Design review of the part built by this model. Coordinates are the model's own, in mm. A direction names the side the tool comes from. Coordinates: 2 decimals unless noted, no trailing zeros. Write each loop counter-clockwise with the first axis right and the second up, starting at its lowest first coordinate (ties: lowest second). Pieces come first, ordered by that corner, then holes.
Q1. Take a section at A-A, the plane y = 42.5. Write out the cut boundary in (x, z).
Q2. For L1, parallel to Y at x = -8.5, z = -21; L2, parallel to Y at x = -0.5, z = 22; L3, parallel to X at y = 58.25, z = -7.5, list the stretches that pass through material, from the lowest coordinate up.
Q3. For faces 1 (the flat face through (-58, 46.058, 0)), 2 (the cylindrical face through (-25.977, 46.71, -0.66)), 3 (the flat face through (-59.366, 36.9, 1.1)), 4 (the flat face through (-46, 33, -13.5)), list the 3-axis set-ups (+Z, -Z, +X, -X, +Y, -Y) from which the entire face can be reached by the end or side of a thin tool; tool diameter is ignored.
Q4. Take a section at C-C, the plane y = 50.25. Write out the cut boundary in (x, z).
Q5. Take a section at D-D, the plane x = -22.5. Write out the cut boundary in (y, z), plus the area to 3 significant figures.
Q6. For pin 1 Ø4.5 at (x, z) = (-51, 2) entering from -Y; pin 2 Ø8 at (x, y) = (-6, 44) entering from -Z; pin 3 Ø2.5 at (x, y) = (-58, 42.5) entering from +Z, all flat-tipped, find the tip position at first contact; note any pin that passes through.
Q7. The part is to be moulded in two halves that separate along Z. For faces 5 (the flat face through (-44, 33, 16.771)), 6 (the flat face through (-57.116, 36.9, 2.1)), 7 (the flat face through (-58, 42, -12)), say which applies: released by +Z, released by -Z, zero draft, split by the parting line, or undercut.
from build123d import *

# Parameters (mm, degrees)
SKETCH1_R               = 50
BOSS_EXTRUDE1_DEPTH     = 7.5
SKETCH1_2_R             = 50
BOSS_EXTRUDE2_DEPTH     = 90
SKETCH2_W               = 7.5
SKETCH2_H               = 90
BOSS_EXTRUDE3_DEPTH     = 40
SKETCH4_R               = 100
BOSS_EXTRUDE4_DEPTH     = 2.5
SKETCH7_W               = 90
SKETCH7_H               = 50
BOSS_EXTRUDE9_DEPTH     = 7.5
CUT_EXTRUDE1_REACH      = 263.25
SKETCH14_W              = 95
SKETCH14_H              = 90
BOSS_EXTRUDE13_DEPTH    = 3
BOSS_EXTRUDE14_DEPTH    = 5
SKETCH17_W              = 70.898930346
SKETCH17_H              = 90
CUT_EXTRUDE3_DEPTH      = 5
CUT_EXTRUDE3_DEPTH_BACK = 1
CHAMFER3_SIZE           = 2
CHAMFER3_SIZE2          = 57.272506566
SCALE1_SCALE            = 0.3
CUT_EXTRUDE4_REACH      = 4.25
SKETCH19_R              = 1.75


with BuildPart() as part:
    # Sketch1 → Boss-Extrude1 (new body)
    with BuildSketch(Plane(origin=(0, 0, 0), x_dir=(1, 0, 0), z_dir=(0, 1, 0))):
        with BuildLine():
            Line((-50, 55.901699437), (-170, 55.901699437))
            Line((-170, 55.901699437), (-170, -55.901699437))
            Line((-170, -55.901699437), (-50, -55.901699437))
            ThreePointArc((-50, -55.901699437), (75, 0), (-50, 55.901699437))
        make_face()
        Circle(SKETCH1_R, mode=Mode.SUBTRACT)
        with BuildLine():
            Line((-95, -45), (-135, -45))
            ThreePointArc((-135, -45), (-142.071067812, -42.071067812), (-145, -35))
            Line((-145, -35), (-145, 35))
            ThreePointArc((-145, 35), (-142.071067812, 42.071067812), (-135, 45))
            Line((-135, 45), (-95, 45))
            ThreePointArc((-95, 45), (-80.857864376, 39.142135624), (-75, 25))
            Line((-75, 25), (-75, -25))
            ThreePointArc((-75, -25), (-80.857864376, -39.142135624), (-95, -45))
        make_face(mode=Mode.SUBTRACT)
    extrude(amount=BOSS_EXTRUDE1_DEPTH)

    # Sketch1_2 → Boss-Extrude2 (add)
    with BuildSketch(Plane(origin=(0, 0, 0), x_dir=(1, 0, 0), z_dir=(0, 1, 0))):
        Circle(SKETCH1_2_R)
    extrude(amount=BOSS_EXTRUDE2_DEPTH)

    # Sketch2 → Boss-Extrude3 (add)
    with BuildSketch(Plane(origin=(0, 7.5, 0), x_dir=(1, 0, 0), z_dir=(0, 1, 0))):
        with Locations((-157.5, 0)):
            Rectangle(SKETCH2_W, SKETCH2_H)
    extrude(amount=BOSS_EXTRUDE3_DEPTH)

    # Sketch4 → Boss-Extrude4 (add)
    with BuildSketch(Plane(origin=(0, 90, 0), x_dir=(1, 0, 0), z_dir=(0, 1, 0))):
        Circle(SKETCH4_R)
    extrude(amount=BOSS_EXTRUDE4_DEPTH)

    # Sketch7 → Boss-Extrude9 (add)
    with BuildSketch(Plane(origin=(-162.32329818, 43.49439666, 0), x_dir=(0, 0, 1), z_dir=(-0.965925826, 0.258819045, 0))):
        with Locations((0, 29.146905726)):
            Rectangle(SKETCH7_W, SKETCH7_H)
    extrude(amount=-BOSS_EXTRUDE9_DEPTH)

    # Sketch3 → Cut-Extrude1 (cut, up to next)
    with BuildSketch(Plane.ZY.offset(161.25), mode=Mode.PRIVATE) as cut_extrude1_sk1:
        Polygon((35, 46), (40, 41), (40, 21), (35, 16), (-35, 16), (-40, 21), (-40, 41), (-35, 46), align=None)
    cut_extrude1_tool1 = extrude(cut_extrude1_sk1.sketch, amount=-CUT_EXTRUDE1_REACH, mode=Mode.PRIVATE) & part.part
    add(cut_extrude1_tool1.solids().sort_by_distance((-161.25, 31, 0))[0], mode=Mode.SUBTRACT)

    # Sketch14 → Boss-Extrude13 (add)
    with BuildSketch(Plane.XZ.offset(-90)):
        with Locations((-102.34127557, 0)):
            Rectangle(SKETCH14_W, SKETCH14_H)
    extrude(amount=BOSS_EXTRUDE13_DEPTH)

    # Sketch15 → Boss-Extrude14 (add)
    with BuildSketch(Plane(origin=(0, 90, 0), x_dir=(1, 0, 0), z_dir=(0, 1, 0))):
        with BuildLine():
            Line((-92.649878575, 45), (-144.686825896, 45))
            Line((-144.686825896, 45), (-144.686825896, -45))
            Line((-144.686825896, -45), (-92.649878575, -45))
            ThreePointArc((-92.649878575, -45), (-103, 0), (-92.649878575, 45))
        make_face()
    extrude(amount=BOSS_EXTRUDE14_DEPTH)

    # Sketch17 → Cut-Extrude3 (cut, two sides)
    with BuildSketch(Plane(origin=(0, 95, 0), x_dir=(1, 0, 0), z_dir=(0, 1, 0))) as cut_extrude3_sk:
        with Locations((-122.050534827, 0)):
            Rectangle(SKETCH17_W, SKETCH17_H)
    extrude(amount=CUT_EXTRUDE3_DEPTH, mode=Mode.SUBTRACT)
    extrude(cut_extrude3_sk.sketch, amount=-CUT_EXTRUDE3_DEPTH_BACK, mode=Mode.SUBTRACT)

    # Chamfer3
    chamfer3_edges = [part.edges().sort_by_distance(p)[0] for p in [
        (-54.84127557, 87, 0),
    ]]
    chamfer3_side = [part.faces().sort_by_distance(p)[0] for p in [
        (-54.84127557, 88.5, 0),
    ]]
    chamfer(chamfer3_edges, length=CHAMFER3_SIZE, length2=CHAMFER3_SIZE2, reference=chamfer3_side[0])


with BuildPart() as part_1:
    # Scale1: scaled about (-15.701446572, 46.083241644, 0)
    add(part.part.scale(SCALE1_SCALE).moved(Location((-10.9910126, 32.258269151, 0))))

    # Sketch19 → Cut-Extrude4 (cut, up to next)
    with BuildSketch(Plane(origin=(0, 34.50826915, 0), x_dir=(1, 0, 0), z_dir=(0, 1, 0)), mode=Mode.PRIVATE) as cut_extrude4_sk1:
        with Locations((-30.491012601, 9.375)):
            Circle(SKETCH19_R)
    cut_extrude4_tool1 = extrude(cut_extrude4_sk1.sketch, amount=-CUT_EXTRUDE4_REACH, mode=Mode.PRIVATE) & part_1.part
    add(cut_extrude4_tool1.solids().sort_by_distance((-30.491013, 34.508269, -9.375))[0], mode=Mode.SUBTRACT)
    # Sketch19 → Cut-Extrude4 (cut, up to next)
    with BuildSketch(Plane(origin=(0, 34.50826915, 0), x_dir=(1, 0, 0), z_dir=(0, 1, 0)), mode=Mode.PRIVATE) as cut_extrude4_sk2:
        with Locations((-30.491012601, -9.375)):
            Circle(SKETCH19_R)
    cut_extrude4_tool2 = extrude(cut_extrude4_sk2.sketch, amount=-CUT_EXTRUDE4_REACH, mode=Mode.PRIVATE) & part_1.part
    add(cut_extrude4_tool2.solids().sort_by_distance((-30.491013, 34.508269, 9.375))[0], mode=Mode.SUBTRACT)


solid = part_1.part
Responses:
1. outline: (-59.37, -13.5) - (-57.12, -13.5) - (-57.12, -12) - (-59.37, -12) - close; (-59.37, 12) - (-57.12, 12) - (-57.12, 13.5) - (-59.37, 13.5) - close; circle Ø30 at (-10.99, 0)
2. L1: y = 32.26 to 34.51, 59.26 to 60.01
2. L2: y = 59.26 to 60.01
2. L3: x = -56.22 to -53.89, -23.98 to 2
3. face 1: -X
3. face 2: none
3. face 3: +Z, -Z, -X, +Y
3. face 4: -Y
4. outline: (-58.36, -13.5) - (-56.03, -13.5) - (-56.03, 13.5) - (-58.36, 13.5) - close; circle Ø30 at (-10.99, 0)
5. outline: (32.26, -19.33) - (34.51, -19.33) - (34.51, -9.62) - (59.26, -9.62) - (59.26, -27.7) - (60.01, -27.7) - (60.01, 27.7) - (59.26, 27.7) - (59.26, 9.62) - (34.51, 9.62) - (34.51, 19.33) - (32.26, 19.33) - close
5. area: 605 mm2
6. pin 1: stops at y = 58.36
6. pin 2: stops at z = -14.97
6. pin 3: stops at z = 13.5
7. face 5: released by +Z
7. face 6: zero draft
7. face 7: undercut
